from build123d import *

# Parameters (mm, degrees)
EXTRUDE_THIN1_DEPTH = 15
FILLET1_R           = 4
SKETCH6_R           = 2
SKETCH6_W           = 20
SKETCH6_H           = 10
CUT_EXTRUDE4_DEPTH  = 29.185938934


with BuildPart() as part:
    # Sketch1 → Extrude-Thin1 (new body, symmetric)
    with BuildSketch(Plane.XY):
        with BuildLine():
            Line((27.085573469, 12.435938934), (12.085573469, 12.435938934))
            Line((12.085573469, 12.435938934), (12.085573469, 4.435938934))
            ThreePointArc((12.085573469, 4.435938934), (0.132124352, -12.75), (-11.821324764, 4.435938934))
            Line((-11.821324764, 4.435938934), (-11.821324764, 12.435938934))
            Line((-11.821324764, 12.435938934), (-26.821324764, 12.435938934))
            Line((-26.821324764, 12.435938934), (-26.821324764, 9.435938934))
            Line((-26.821324764, 9.435938934), (-14.821324764, 9.435938934))
            Line((-14.821324764, 9.435938934), (-14.821324764, 4.945387703))
            ThreePointArc((-14.821324764, 4.945387703), (0.132124352, -15.75), (15.085573469, 4.945387703))
            Line((15.085573469, 4.945387703), (15.085573469, 9.435938934))
            Line((15.085573469, 9.435938934), (27.085573469, 9.435938934))
            Line((27.085573469, 9.435938934), (27.085573469, 12.435938934))
        make_face()
    extrude(amount=EXTRUDE_THIN1_DEPTH, both=True)

    # Fillet1
    fillet1_edges = [part.edges().sort_by_distance(p)[0] for p in [
        (15.085573469, 9.435938934, 0),
        (-14.821324764, 9.435938934, 0),
    ]]
    fillet(fillet1_edges, radius=FILLET1_R)

    # Sketch6 → Cut-Extrude4 (cut, through all)
    with BuildSketch(Plane(origin=(0, 12.435938934, 0), x_dir=(1, 0, 0), z_dir=(0, 1, 0))):
        with Locations((-19.321324764, 0)):
            Circle(SKETCH6_R)
        with Locations((19.321324764, 0)):
            Circle(SKETCH6_R)
        Rectangle(SKETCH6_W, SKETCH6_H)
    extrude(amount=-CUT_EXTRUDE4_DEPTH, mode=Mode.SUBTRACT)


solid = part.part
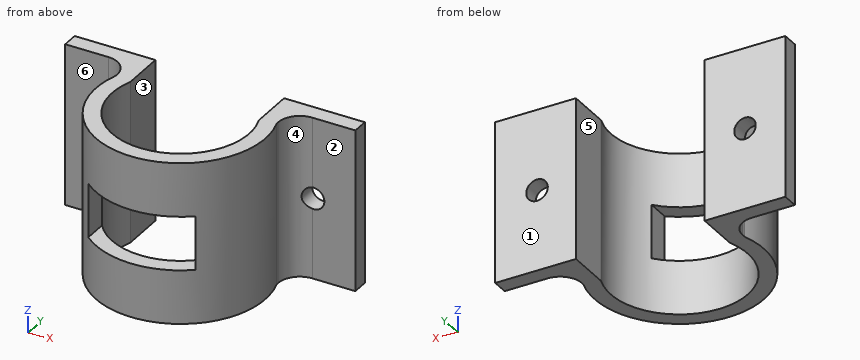
Geometry check sheet. Reference: the model listing, model coordinates, mm. Face numbers are marked on the shaded views. A direction names the side the tool comes from. Round coordinates to 2 decimals unless told otherwise and drop trailing zeros. Write each loop counter-clockwise with the first axis right and the second up, starting at its lowest first coordinate (ties: lowest second). Pieces come first, ordered by that corner, then holes.
Item 1: Section check D-D (z = -11). Record the boundary of the cut face in (x, y).
Determined:
outline: (-26.82, 9.44) - (-18.82, 9.44) arc R4 cw to (-14.82, 5.44) - (-14.82, 4.95) arc R15.75 ccw (long way) to (15.09, 4.95) - (15.09, 5.44) arc R4 cw to (19.09, 9.44) - (27.09, 9.44) - (27.09, 12.44) - (12.09, 12.44) - (12.09, 4.44) arc R12.75 cw (long way) to (-11.82, 4.44) - (-11.82, 12.44) - (-26.82, 12.44) - close
Item 2: Mould release check, pull along X, two halves, no side actions. Record for the marked faces 3, 4, 5 and 6: +X half, -X half, draft (parallel to the pull), parting line (faces both ways), or undercut.
Determined:
face 3: undercut
face 4: +X half
face 5: undercut
face 6: draft
Item 3: Material ranges on line 1 along X through (y, z) = (10.25, 0); line 2 along X through (y, z) = (0, 3.75); line 3 along X through (y, z) = (-1.5, 0.5), recorded low to high.
Determined:
line 1: x = -26.82 to -21.32, -17.32 to -11.82, 12.09 to 17.32, 21.32 to 27.09
line 2: x = -15.62 to -12.62, 12.88 to 15.88
line 3: x = -15.55 to -12.53, 12.79 to 15.81
Item 4: Section check A-A (z = 0). Record the boundary of the cut face in (x, y).
Determined:
outline: (-26.82, 9.44) - (-21.32, 9.44) - (-21.32, 12.44) - (-26.82, 12.44) - close; (-17.32, 9.14) arc R4 cw to (-14.82, 5.44) - (-14.82, 4.95) arc R15.75 ccw to (-10, -12.06) - (-10, -7.74) arc R12.75 cw to (-11.82, 4.44) - (-11.82, 12.44) - (-17.32, 12.44) - close; (10, -12.28) arc R15.75 ccw to (15.09, 4.95) - (15.09, 5.44) arc R4 cw to (17.32, 9.03) - (17.32, 12.44) - (12.09, 12.44) - (12.09, 4.44) arc R12.75 cw to (10, -8.07) - close; (21.32, 9.44) - (27.09, 9.44) - (27.09, 12.44) - (21.32, 12.44) - close
Item 5: Go/stop test with flat-tipped pins: pin 1 Ø9 at (x, z) = (21.5, -1.5) entering from -Y; pin 2 Ø4 at (y, z) = (-4, 9.5) entering from +X; pin 3 Ø5 at (y, z) = (-5, 2) entering from +X. Record where each tip stops, or that it passes through.
Determined:
pin 1: stops at y = 8.85
pin 2: stops at x = 15.75
pin 3: stops at x = 15.68
Item 6: Section check C-C (x = -5.5). Record the boundary of the cut face in (y, z), plus the area to 3 significant figures.
Determined:
outline: (-14.71, -15) - (-11.44, -15) - (-11.44, -5) - (-14.71, -5) - close; (-14.71, 5) - (-11.44, 5) - (-11.44, 15) - (-14.71, 15) - close
area: 65.4 mm2
Item 7: Section check B-B (y = 0). Record the boundary of the cut face in (x, z), plus the area to 3 significant figures.
Determined:
outline: (-15.62, -15) - (-12.62, -15) - (-12.62, 15) - (-15.62, 15) - close; (12.88, -15) - (15.88, -15) - (15.88, 15) - (12.88, 15) - close
area: 180 mm2
Item 8: Access from +Z, -Z, +X, -X, +Y, -Y to the whole of each face (thin tool, end or side, straight path). Record for the marked faces 1 and 2.
Determined:
face 1: +Z, -Z, +X, -X, +Y
face 2: +Z, -Z, +X, -Y
